Could you check a few things on this model? Use its own coordinates, in mm. Round coordinates to 2 decimals unless told otherwise and drop trailing zeros. Loops run counter-clockwise (first coordinate to the right, second up) from the corner with the lowest first, then second, coordinate; pieces in that order, holes last. Notation, with made-up numbers: (65, -5.75) -> (76, -5.75) arc R13 cw to (76, 8.25) -> close; hole circle Ø1 at (56, -3). An arc over 180 degrees is marked (long way). One line per item, written item: value.
```python
from build123d import *

# Parameters (mm, degrees)
SKETCH1_R           = 1.5
BOSS_EXTRUDE1_DEPTH = 1.5
CUT_EXTRUDE1_REACH  = 65.955
SKETCH2_W           = 87
SKETCH2_H           = 56


with BuildPart() as part:
    # Sketch1 → Boss-Extrude1 (new, symmetric)
    with BuildSketch(Plane(origin=(0, 0, 0), x_dir=(1, 0, 0), z_dir=(0, 1, 0))):
        with BuildLine():
            Line((48, -32.5), (-48, -32.5))
            ThreePointArc((-48, -32.5), (-52.949747468, -30.449747468), (-55, -25.5))
            Line((-55, -25.5), (-55, 25.5))
            ThreePointArc((-55, 25.5), (-52.949747468, 30.449747468), (-48, 32.5))
            Line((-48, 32.5), (48, 32.5))
            ThreePointArc((48, 32.5), (52.949747468, 30.449747468), (55, 25.5))
            Line((55, 25.5), (55, -25.5))
            ThreePointArc((55, -25.5), (52.949747468, -30.449747468), (48, -32.5))
        make_face()
        with Locations(Location((-47.05, 24.27, 0), (0, 0, 270))):
            Circle(SKETCH1_R, mode=Mode.SUBTRACT)
        with Locations(Location((-47.05, -24.27, 0), (0, 0, 270))):
            Circle(SKETCH1_R, mode=Mode.SUBTRACT)
        with Locations(Location((47.05, -24.27, 0), (0, 0, 270))):
            Circle(SKETCH1_R, mode=Mode.SUBTRACT)
        with Locations(Location((47.05, 24.27, 0), (0, 0, 270))):
            Circle(SKETCH1_R, mode=Mode.SUBTRACT)
    extrude(amount=BOSS_EXTRUDE1_DEPTH, both=True)

    # Sketch2 → Cut-Extrude1 (cut, up to next)
    with BuildSketch(Plane(origin=(0, 1.5, 0), x_dir=(1, 0, 0), z_dir=(0, 1, 0)), mode=Mode.PRIVATE) as cut_extrude1_sk1:
        Rectangle(SKETCH2_W, SKETCH2_H)
    cut_extrude1_tool1 = extrude(cut_extrude1_sk1.sketch, amount=-CUT_EXTRUDE1_REACH, mode=Mode.PRIVATE) & part.part
    add(cut_extrude1_tool1.solids().sort_by_distance((0, 1.5, 0))[0], mode=Mode.SUBTRACT)


solid = part.part
```
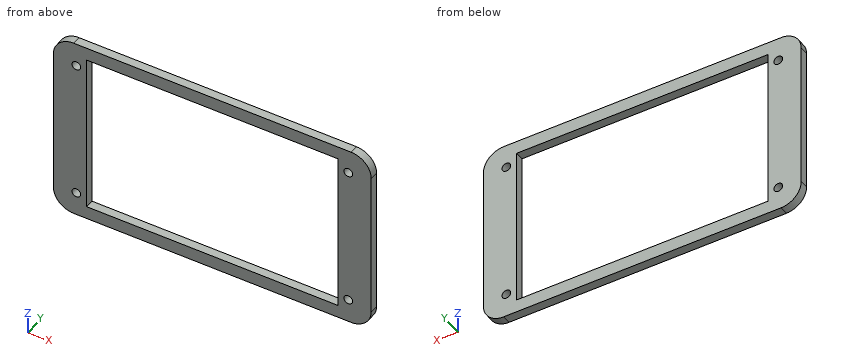
(1) Imagine slicing it at C-C on y = -0.75. Write out the boundary of the cut face in (x, z), then the cut area to 3 significant figures.
Results below:
outline: (-55, -25.5) arc R7 ccw to (-48, -32.5) -> (48, -32.5) arc R7 ccw to (55, -25.5) -> (55, 25.5) arc R7 ccw to (48, 32.5) -> (-48, 32.5) arc R7 ccw to (-55, 25.5) -> close; hole circle Ø3 at (-47.05, -24.27); hole circle Ø3 at (-47.05, 24.27); hole (-43.5, -28) -> (43.5, -28) -> (43.5, 28) -> (-43.5, 28) -> close; hole circle Ø3 at (47.05, -24.27); hole circle Ø3 at (47.05, 24.27)
area: 2,210 mm²
(2) Imagine slicing it at D-D on x = 42. Write out the boundary of the cut face in (y, z), then the cut area to 3 significant figures.
Results below:
outline: (-1.5, -32.5) -> (1.5, -32.5) -> (1.5, -28) -> (-1.5, -28) -> close; (-1.5, 28) -> (1.5, 28) -> (1.5, 32.5) -> (-1.5, 32.5) -> close
area: 27.0 mm²
(3) Please list where these lines run through material, in increasing order: L1, parallel to X at y = -0.5, z = 24.27; L2, parallel to X at y = -1.4, z = -14; L3, parallel to Z at x = -8, y = -0.3.
Results below:
L1: x = -55 to -48.55, -45.55 to -43.5, 43.5 to 45.55, 48.55 to 55
L2: x = -55 to -43.5, 43.5 to 55
L3: z = -32.5 to -28, 28 to 32.5
(4) Imagine slicing it at B-B on z = -24.27. Write out the boundary of the cut face in (x, y).
Results below:
outline: (-55, -1.5) -> (-48.55, -1.5) -> (-48.55, 1.5) -> (-55, 1.5) -> close; (-45.55, -1.5) -> (-43.5, -1.5) -> (-43.5, 1.5) -> (-45.55, 1.5) -> close; (43.5, -1.5) -> (45.55, -1.5) -> (45.55, 1.5) -> (43.5, 1.5) -> close; (48.55, -1.5) -> (55, -1.5) -> (55, 1.5) -> (48.55, 1.5) -> close
(5) Imagine slicing it at A-A on z = 13. Write out the boundary of the cut face in (x, y).
Results below:
outline: (-55, -1.5) -> (-43.5, -1.5) -> (-43.5, 1.5) -> (-55, 1.5) -> close; (43.5, -1.5) -> (55, -1.5) -> (55, 1.5) -> (43.5, 1.5) -> close
